The figure shows three views and two pictorial views of one solid part (mm, origin at its lowest corner). Answer the questions. Round coordinates to 2 decimals unless told otherwise and drop trailing zeros. Order: outer loops, then holes, each group sorted by start corner. A loop starts at its lowest first (then second) coordinate and runs counter-clockwise, first axis right, second up. Notation, with made-up numbers: (43, 27) -> (70, 27) arc R19 ccw to (70, 47) -> close; hole circle Ø6 at (62, 18). An arc over 180 degrees is marked (long way). Return JSON: item names as keys, results as strings. Group by question number.
(1) This flat-tipped pin is pushed along its axis until it touches: pin 1 (2.5 mm diameter, centred on x = 37, z = 2, fed in from -Y). Where does it stop, or does it pass through?
(2) Consider line 1 (X direction, y = 1.75, z = 2.3); line 2 (X direction, y = 2.75, z = 3.6) (3 decimals); line 3 (Y direction, x = 20.5, z = 0.8). Determine where each line is inside the solid, lowest interval first. Write a range as [from, to].
(3) The part is cut by section C-C (x = 32.5). Determine the outline of the cut face in (y, z), plus the area to 3 significant figures.
(4) Determine the mould class of the marked faces 1 and 2 for opening direction X: +X half, -X half, draft (parallel to the pull), parting line (faces both ways), or undercut.
(5) The part is cut by section B-B (z = 0.5). Determine the outline of the cut face in (x, y), plus the area to 3 significant figures.
(6) The part is cut by section A-A (y = 4.5). Determine the outline of the cut face in (x, z), plus the area to 3 significant figures.
(7) The part is cut by section D-D (y = 7.25). Determine the outline of the cut face in (x, z).
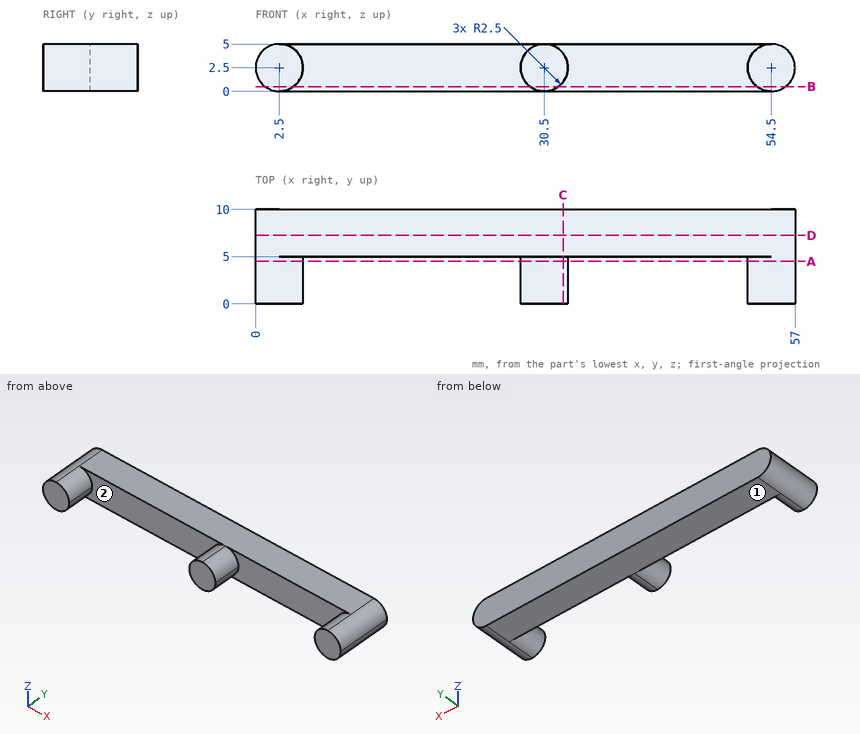
Answer below:
{
 "1": {"pin 1": "stops at y = 5"},
 "2": {"line 1": "x = [0.01, 4.99], [28.01, 32.99], [52.01, 56.99]", "line 2": "x = [0.255, 4.745], [28.255, 32.745], [52.255, 56.745]", "line 3": "y = [5, 10]"},
 "3": {"outline": "(0, 1) -> (5, 1) -> (5, 0) -> (10, 0) -> (10, 5) -> (5, 5) -> (5, 4) -> (0, 4) -> close", "area": "40.0 mm²"},
 "4": {"face 1": "draft", "face 2": "undercut"},
 "5": {"outline": "(1, 0) -> (4, 0) -> (4, 5) -> (29, 5) -> (29, 0) -> (32, 0) -> (32, 5) -> (53, 5) -> (53, 0) -> (56, 0) -> (56, 10) -> (1, 10) -> close", "area": "320 mm²"},
 "6": {"outline": "circle Ø5 at (2.5, 2.5); circle Ø5 at (30.5, 2.5); circle Ø5 at (54.5, 2.5)", "area": "58.9 mm²"},
 "7": {"outline": "(2.5, 0) -> (54.5, 0) arc R2.5 ccw to (54.5, 5) -> (2.5, 5) arc R2.5 ccw to start"}
}
